Autodesk Inventor part; units mm, degrees
ref_plane "YZ Plane" through (0, 0, 0) normal (1, 0, 0) x (0, 1, 0)
ref_plane "XZ Plane" through (0, 0, 0) normal (0, 1, 0) x (-1, 0, 0)
ref_plane "XY Plane" through (0, 0, 0) normal (0, 0, 1) x (1, 0, 0)
sketch "Boceto1" plane through (0, 0, 0) normal (0, 1, 0) x (-1, 0, 0)
  line L0 (0, 0) -> (100, 0)
  line L1 (100, 0) -> (100, 250)
  line L2 (100, 250) -> (30, 250)
  line L3 (0, 0) -> (0, 190)
  circle A0 centre (0, 190) radius 30
  line L4 (30, 250) -> (30, 190)
  line L5 (0, 40) -> (100, 40)
  line L6 (-30, 190) -> (-30, 250)
  line L7 (-30, 250) -> (-100, 250)
  line L8 (-100, 250) -> (-100, 0)
  line L9 (-108.7956, 0) -> (-108.7956, 100)
  line L10 (-108.7956, 100) -> (100, 100)
  line L11 (100, 0) -> (100, -250)
  line L12 (100, -250) -> (30, -250)
  circle A1 centre (0, -190) radius 30
  line L13 (30, -250) -> (30, -190)
  line L14 (-30, -190) -> (-30, -250)
  line L15 (-30, -250) -> (-100, -250)
  line L16 (-100, -250) -> (-100, 0)
  point P0 (0, -40)
  point P1 (100, -40)
  point P2 (100, -100)
  dimension "d0" = 100
  dimension "d1" = 250
  dimension "d2" = 70
  dimension "d3" = 190
  dimension "d4" = 60
  dimension "d6" = 70
  dimension "d7" = 100
extrude "Extrusión1" add sketch "Boceto1" along normal blind 25 contours L3 L5 L1 L0 | L0 L11 L12 L13 A1 L14 L15 L16 L8 L10 L3 | L3 L10 L1 L5 | L10 L8 L7 L6 A0 L3 | L3 A0 L4 L2 L1 L10
sketch "Boceto2" plane through (0, 25, 0) normal (0, 1, 0) x (1, 0, 0)
  circle A0 centre (0, 0) radius 40
  line L0 (100, -250) -> (100, 250)
  line L1 (100, 0) -> (100, -100)
  line L2 (100, -100) -> (-100, -100)
  line L3 (-100, 250) -> (-100, -250)
  line L4 (-40, 0) -> (40, 0)
  line L5 (100, 100) -> (-100, 100)
  line L6 (0, -40) -> (-100, -40)
  line L7 (0, 40) -> (-100, 40)
  dimension "d10" = 80
  dimension "d11" = 100
extrude "Extrusión2" add sketch "Boceto2" along normal blind 35 contours A0 L7 L3 L5 L0 L2 L6
sketch "Boceto3" plane through (0, 25, 0) normal (0, 1, 0) x (1, 0, 0)
  line L0 (-100, 40) -> (0, 40)
  circle A0 centre (0, 0) radius 40
  line L1 (0, 40) -> (-100, 40)
  line L2 (0, -40) -> (-100, -40)
  line L3 (-100, 40) -> (-100, -40)
  line L4 (-100, 40) -> (-100, -40)
extrude "Extrusión3" cut sketch "Boceto3" against normal blind 5
sketch "Boceto4" plane through (0, 60, 0) normal (0, 1, 0) x (1, 0, 0)
  line L0 (100, 100) -> (-100, 100)
  line L1 (100, -100) -> (-100, -100)
  line L2 (100, 100) -> (70, 100)
  line L3 (70, 100) -> (70, -100)
  line L4 (70, -100) -> (100, -100)
  line L5 (100, -100) -> (100, 100)
  point P0 (0, 0)
  dimension "d16" = 30
extrude "Extrusión4" add sketch "Boceto4" along normal blind 190
sketch "Boceto5" plane through (70, 60, -100) normal (-1, 0, 0) x (0, 0, 1)
  line L0 (200, 0) -> (0, 0)
  line L1 (100, 0) -> (100, 90)
  circle A0 centre (100, 90) radius 50
  point P0 (100, -60)
  dimension "d19" = 90
  dimension "d20" = 100
extrude "Extrusión5" cut sketch "Boceto5" against normal blind 190
fillet "Empalme1" radius 100 2 edges at (85, 250, -100) (85, 250, 100)
sketch "Boceto6" plane through (-100, 0, -250) normal (-1, 0, 0) x (0, 0, 1)
  line L0 (150, 25) -> (150, 60)
  line L1 (150, 60) -> (150, 55)
  line L2 (150, 25) -> (0, 25)
  line L3 (150, 55) -> (0, 25)
  line L4 (250, 88.3729) -> (250, -17.9249)
  line L5 (350, 25) -> (350, 60)
  line L6 (350, 25) -> (500, 25)
  line L7 (350, 55) -> (500, 25)
  point P0 (250, 0)
  dimension "d24" = 5
extrude "Extrusión6" add sketch "Boceto6" against normal blind 200
sketch "Boceto7" plane through (0, 25, -190) normal (0, -1, 0) x (1, 0, 0)
  line L0 (30, -60) -> (30, 0)
  circle A0 centre (0, 0) radius 30
  line L1 (30, 0) -> (30, -60)
  line L2 (-30, -60) -> (30, -60)
  line L3 (-30, -60) -> (-100, -60)
  line L4 (30, -60) -> (-30, -60)
  line L5 (-30, -60) -> (-30, 0)
  line L6 (105.1195, 190) -> (-118.3663, 190)
  line L7 (30, 440) -> (30, 380)
  circle A1 centre (0, 380) radius 30
  line L8 (-30, 440) -> (30, 440)
  line L9 (-30, 440) -> (-30, 380)
  point P0 (0, 190)
extrude "Extrusión7" cut sketch "Boceto7" against normal blind 200
The model under review builds one solid part; all positions refer to its coordinate system, in mm. A direction names the side the tool comes from. Round coordinates to 2 decimals unless told otherwise and drop trailing zeros. Order: outer loops, then holes, each group sorted by start corner. A loop starts at its lowest first (then second) coordinate and runs counter-clockwise, first axis right, second up. Notation, with made-up numbers: (54, -11.75) -> (77, -11.75) arc R16 cw to (77, 5.25) -> close; hole circle Ø11 at (48, -4.5). An arc over 180 degrees is marked (long way). Return JSON: item names as keys, results as strings.
1. For L1, parallel to Y at x = 84, z = 0; L2, parallel to Y at x = 56.5, z = -92.5; L3, parallel to X at y = 98.5, z = -6, list the stretches that pass through material, from the lowest coordinate up. Write a range as [from, to].
Answer block:
{"L1": "y = [0, 100], [200, 250]", "L2": "y = [0, 60]", "L3": "x = [70, 100]"}
2. Take a section at C-C (z = 138.5). Write out the cut boundary in (x, y).
Answer block:
{"outline": "(-100, 0) -> (100, 0) -> (100, 47.3) -> (-100, 47.3) -> close"}
3. Take a section at A-A (x = -35.5). Write out the cut boundary in (y, z).
Answer block:
{"outline": "(0, -250) -> (25, -250) -> (55, -100) -> (60, -100) -> (60, -40) -> (20, -40) -> (20, 40) -> (60, 40) -> (60, 100) -> (55, 100) -> (25, 250) -> (0, 250) -> close"}
4. The part is to be moulded in two halves that separate along Z. For faces 5 (the face through (-30, 14, 220)), 6 (the face through (-49, 40, 40)), 7 (the face through (84.79, 101.19, -10.84)), 8 (the face through (0.66, 21.209, -160.007)), say which applies: +Z half, -Z half, draft (parallel to the pull), parting line (faces both ways), or undercut.
Answer block:
{"face 5": "draft", "face 6": "undercut", "face 7": "undercut", "face 8": "-Z half"}
5. For faces 1 (the face through (-16, 60, -46)), 2 (the face through (75, 95, 100)), 3 (the face through (30, 14, 220)), 4 (the face through (39.99, 39.72, -0.88)), list the 3-axis set-ups (+Z, -Z, +X, -X, +Y, -Y) from which the entire face can be reached by the end or side of a thin tool; tool diameter is ignored.
Answer block:
{"face 1": "+Z, -Z, -X, +Y", "face 2": "+Z, +X, -X, +Y", "face 3": "+Z, +Y, -Y", "face 4": "-X, +Y"}
6. Take a section at B-B (y = 131). Write out the cut boundary in (x, z), then the cut area to 3 significant figures.
Answer block:
{"outline": "(70, -100) -> (100, -100) -> (100, -46.25) -> (70, -46.25) -> close; (70, 46.25) -> (100, 46.25) -> (100, 100) -> (70, 100) -> close", "area": "3,230 mm²"}
7. Take a section at D-D (x = 48). Write out the cut boundary in (y, z).
Answer block:
{"outline": "(0, -250) -> (25, -250) -> (55, -100) -> (60, -100) -> (60, 100) -> (55, 100) -> (25, 250) -> (0, 250) -> close"}
8. Insertion check: P1, Ø1.5, axis at y = 120, z = -48.5, coming from the -X side; P2, Ø8, axis at x = -15.5, z = -137.5, coming from the +Y side; P3, Ø4, axis at x = 36, z = -90.5, coming from the +Y side. Each pin has a flat end and moves straight along its axis. Give the tip position at first contact, or say it passes through.
Answer block:
{"P1": "stops at x = 70", "P2": "stops at y = 48.3", "P3": "stops at y = 60"}
